Answer from the drawing. Dimensions are ordinates in mm from the lowest x, y and z of the part. Coordinates: 2 decimals unless noted, no trailing zeros. Write each loop counter-clockwise with the first axis right and the second up, starting at its lowest first coordinate (ties: lowest second). Pieces come first, ordered by that corner, then holes.
1) The part is cut by section A-A (x = 50.8). Determine the outline of the cut face in (y, z) (3 decimals).
2) The part is cut by section C-C (z = 127). Determine the outline of the cut face in (x, y), then the cut area to 3 significant figures.
3) The part is cut by section B-B (y = 50.8). Determine the outline of the cut face in (x, z).
4) Determine the mould class of the marked faces 1, 2 and 3 for opening direction Y: +Y half, -Y half, draft (parallel to the pull), parting line (faces both ways), or undercut.
5) Find the intervals of material crossed by line 1 (Y direction, x = 50.8, z = 110.5); line 2 (Z direction, x = 50.8, y = 99.5); line 3 (Z direction, x = 49.5, y = 78), in increasing order.
6) The part is cut by section D-D (z = 73.5). Determine the outline of the cut face in (x, y), then the cut area to 3 significant figures.
7) Each of these flat-tipped pins is pushed along its axis until it touches: pin 1 Ø1.5 at (y, z) = (47, 96.5) entering from +X; pin 2 Ø4 at (x, z) = (16, 43.5) entering from -Y; pin 3 Ø2 at (y, z) = (68, 113) entering from +X; pin 4 Ø16.5 at (x, z) = (50.8, 127) entering from +Y. Where does it stop, or does it pass through?
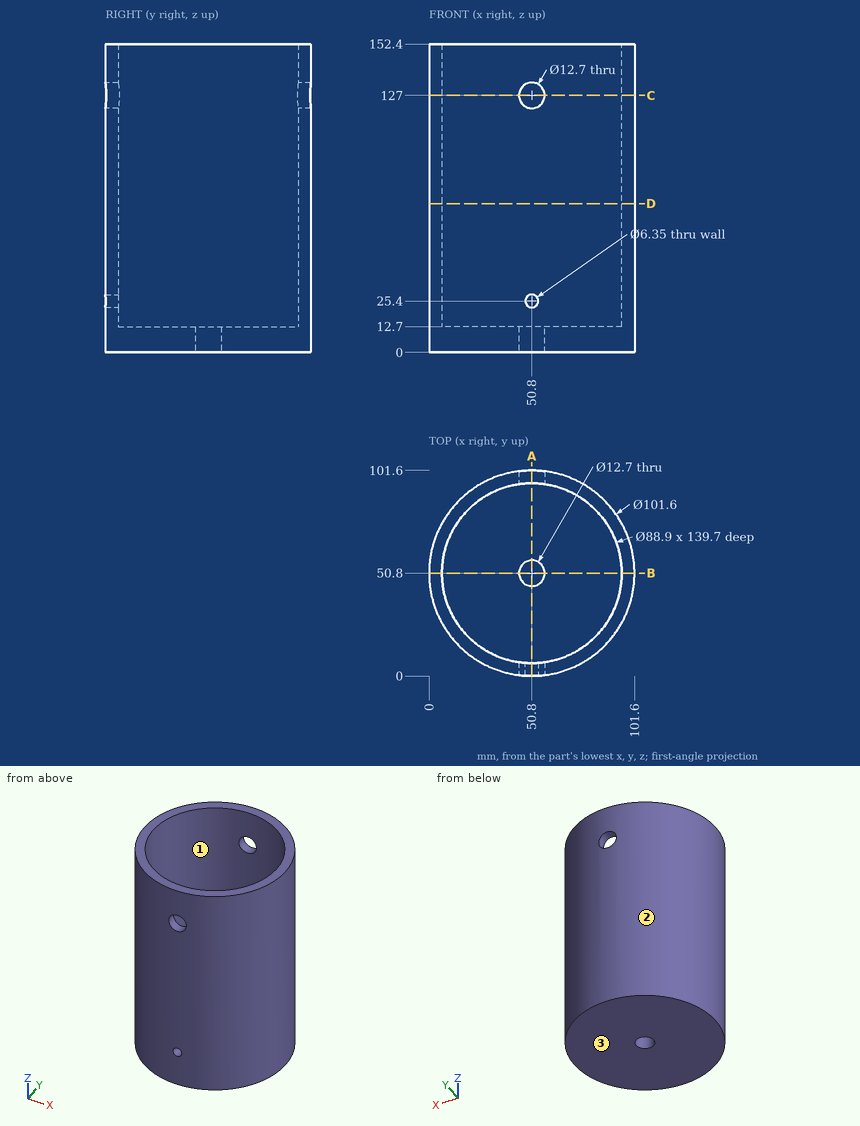
Reported:
1. outline: (0, 0) - (44.45, 0) - (44.45, 12.7) - (6.35, 12.7) - (6.35, 22.225) - (0, 22.225) - close; (0, 28.575) - (6.35, 28.575) - (6.35, 120.65) - (0, 120.65) - close; (0, 133.35) - (6.35, 133.35) - (6.35, 152.4) - (0, 152.4) - close; (57.15, 0) - (101.6, 0) - (101.6, 120.65) - (95.25, 120.65) - (95.25, 12.7) - (57.15, 12.7) - close; (95.25, 133.35) - (101.6, 133.35) - (101.6, 152.4) - (95.25, 152.4) - close
2. outline: (44.45, 0.4) - (44.45, 6.81) arc R44.45 cw to (44.45, 94.79) - (44.45, 101.2) arc R50.8 ccw to start; (57.15, 0.4) arc R50.8 ccw to (57.15, 101.2) - (57.15, 94.79) arc R44.45 cw to (57.15, 6.81) - close
2. area: 1,740 mm2
3. outline: (0, 0) - (44.45, 0) - (44.45, 12.7) - (6.35, 12.7) - (6.35, 152.4) - (0, 152.4) - close; (57.15, 0) - (101.6, 0) - (101.6, 152.4) - (95.25, 152.4) - (95.25, 12.7) - (57.15, 12.7) - close
4. face 1: undercut
4. face 2: parting line
4. face 3: draft
5. line 1: y = 0 to 6.35, 95.25 to 101.6
5. line 2: z = 0 to 120.65, 133.35 to 152.4
5. line 3: z = 0 to 12.7
6. outline: circle Ø101.6 at (50.8, 50.8); hole circle Ø88.9 at (50.8, 50.8)
6. area: 1,900 mm2
7. pin 1: stops at x = 101.51
7. pin 2: stops at y = 12.01
7. pin 3: stops at x = 98.95
7. pin 4: stops at y = 101.6
